```python
from build123d import *

# Parameters (mm, degrees)
SKETCH2_R           = 10
BOSS_EXTRUDE1_DEPTH = 12


with BuildPart() as part:
    # Sketch2 → Boss-Extrude1 (new body)
    with BuildSketch(Plane(origin=(0, 0, 0), x_dir=(1, 0, 0), z_dir=(0, 1, 0))):
        Polygon((0, 0), (70, 0), (100, 20), (100, 100), (70, 120), (0, 120), (0, 80), (20, 80), (20, 40), (0, 40), align=None)
        with Locations((20, 100)):
            Circle(SKETCH2_R, mode=Mode.SUBTRACT)
        with Locations((60, 100)):
            Circle(SKETCH2_R, mode=Mode.SUBTRACT)
        with Locations((60, 20)):
            Circle(SKETCH2_R, mode=Mode.SUBTRACT)
        with Locations((20, 20)):
            Circle(SKETCH2_R, mode=Mode.SUBTRACT)
        with Locations((60, 60)):
            Circle(SKETCH2_R, mode=Mode.SUBTRACT)
    extrude(amount=BOSS_EXTRUDE1_DEPTH)


solid = part.part
```
Input: part model. Units: mm. Frame: model coordinates. A direction names the side the tool comes from. Give positions to 0.01 mm unless a question says otherwise; leave off trailing zeros. Order: outer loops, then holes, each group sorted by start corner. A loop starts at its lowest first (then second) coordinate and runs counter-clockwise, first axis right, second up.
1. Cut plane B-B (z = -60). Return loops of the section in (x, y), and give its area (3 significant figures).
Computed:
outline: (20, 0) - (50, 0) - (50, 12) - (20, 12) - close; (70, 0) - (100, 0) - (100, 12) - (70, 12) - close
area: 720 mm2
2. Cut plane A-A (x = 60). Return loops of the section in (y, z), and give its area (3 significant figures).
Computed:
outline: (0, -120) - (12, -120) - (12, -110) - (0, -110) - close; (0, -90) - (12, -90) - (12, -70) - (0, -70) - close; (0, -50) - (12, -50) - (12, -30) - (0, -30) - close; (0, -10) - (12, -10) - (12, 0) - (0, 0) - close
area: 720 mm2
3. Draft query along Z for faces 3 (the face through (85, 6, -10)), 4 (the face through (0, 6, -100)), 5 (the face through (50, 6, -20)). Return one class per face: released by +Z, released by -Z, zero draft, split by the parting line, or undercut.
Computed:
face 3: released by +Z
face 4: zero draft
face 5: undercut
4. Cut plane C-C (y = 3.25). Return loops of the section in (x, z), and give its area (3 significant figures).
Computed:
outline: (0, -120) - (70, -120) - (100, -100) - (100, -20) - (70, 0) - (0, 0) - (0, -40) - (20, -40) - (20, -80) - (0, -80) - close; hole circle Ø20 at (20, -100); hole circle Ø20 at (20, -20); hole circle Ø20 at (60, -100); hole circle Ø20 at (60, -60); hole circle Ø20 at (60, -20)
area: 9,030 mm2
5. Pin query (flat end, axial travel): pin 1 Ø1 at (y, z) = (4.5, -12) entering from +X; pin 2 Ø3.5 at (y, z) = (4, -62) entering from -X; pin 3 Ø1 at (x, y) = (75, 9.5) entering from +Z. Return the tip coordinate at first contact, or that it passes through.
Computed:
pin 1: stops at x = 88.75
pin 2: stops at x = 20
pin 3: stops at z = -3
6. Cut plane D-D (x = 7). Return loops of the section in (y, z), and give its area (3 significant figures).
Computed:
outline: (0, -120) - (12, -120) - (12, -80) - (0, -80) - close; (0, -40) - (12, -40) - (12, 0) - (0, 0) - close
area: 960 mm2
7. Line query: probe 1 along X at (y, z) = (8.25, -100); probe 2 along Z at (x, y) = (60, 7.5); probe 3 along Z at (x, y) = (62, 3.75). Output: solid intervals per line, ascending.
Computed:
probe 1: x = 0 to 10, 30 to 50, 70 to 100
probe 2: z = -120 to -110, -90 to -70, -50 to -30, -10 to 0
probe 3: z = -120 to -109.8, -90.2 to -69.8, -50.2 to -29.8, -10.2 to 0
8. Set-up query: faces 1 (the face through (10, 6, -40)), 2 (the face through (85, 6, -110)). Return all of +Z, -Z, +X, -X, +Y, -Y with unobstructed straight access to the full face (end or side cutting, diameter ignored); none if empty.
Computed:
face 1: -X, +Y, -Y
face 2: -Z, +X, +Y, -Y
